Build history of the part. All positions in model axes, mm. A direction names the side the tool comes from. Coordinates: 2 decimals unless noted, no trailing zeros. Loops run counter-clockwise (first coordinate to the right, second up) from the corner with the lowest first, then second, coordinate; pieces in that order, holes last.
(1) Tool access for faces 5 (the face through (-7, -80, 12)), 6 (the face through (-26, -39.169, 12)), 7 (the face through (-13, -75, 12)): list every direction of +Z, -Z, +X, -X, +Y, -Y with a clear straight run to the whole face (end or side of a thin tool).
(2) Flat gauge pins, fed straight in: P1, Ø1, axis at y = -14, z = 15.5, coming from the +X side; P2, Ø11.5, axis at y = -76.5, z = 9, coming from the -X side; P3, Ø1, axis at x = -16, z = 14, coming from the -Y side; P4, Ø10, axis at x = -37.5, z = 4, coming from the -Y side. Where does each tip first touch, or does it go through?
(3) Slice it at A-A (z = 18.5). Give the number of separate pieces and of enclosed holes in the cut face, and give its area (3 significant figures).
(4) Wall check: L1, parallel to Y at x = -28, z = 23.25; L2, parallel to Y at x = -15.5, z = 7; L3, parallel to Y at x = -58.5, z = 4. Give the ranges that are in metal, low to high.
(5) Two-plate mould, pull along Y, no slides. Class faces 1 (the face through (-27.87, -31.5, 12.32)), 2 (the face through (-23.547, -29.477, 12.325)), 3 (the face through (-39, 0, 12)), 4 (the face through (0, -42, 12)): pulls with the +Y half, pulls with the -Y half, needs draft (parallel to the pull), parting line crosses it, or undercut.
(6) Slice it at B-B (y = -75). Give the cut face in (x, z), and give its area (3 significant figures).
(7) Slice it at C-C (x = -73). Give the cut face in (y, z).
from build123d import *

# Parameters (mm, degrees)
F1_DEPTH = 25
F3_DEPTH = 25


with BuildPart() as f1:
    # F0 (on Top) → F1 (new body)
    with BuildSketch(Plane.XY):
        with BuildLine():
            Line((0, -80), (0, -2))
            ThreePointArc((0, -2), (-0.5857864376, -0.5857864376), (-2, 0))
            Line((-2, 0), (-77.9695956579, 0))
            ThreePointArc((-77.9695956579, 0), (-79.3944371446, -0.5964948388), (-79.9693680385, -2.0301732624))
            Line((-79.9693680385, -2.0301732624), (-79.8235436371, -11.6948759406))
            ThreePointArc((-79.8235436371, -11.6948759406), (-79.2164881491, -13.1000910078), (-77.793597994, -13.6644750587))
            Line((-77.793597994, -13.6644750587), (-53.4198508516, -13.2967154695))
            add(Edge.make_bspline(
                [(-53.4198508516, -13.2967154695), (-47.7391326457, -13.5155175895), (-42.3810972533, -14.1065922457), (-38.542901615, -14.7899318492)],
                knots=[0, 0, 0, 0, 0.162253053, 0.162253053, 0.162253053, 0.162253053], degree=3))
            add(Edge.make_bspline(
                [(-38.542901615, -14.7899318492), (-35.6620781643, -15.3028240882), (-33.637457964, -15.8676938778), (-30.542901615, -17.425809837)],
                knots=[0.162253053, 0.162253053, 0.162253053, 0.162253053, 0.28403486, 0.28403486, 0.28403486, 0.28403486], degree=3))
            add(Edge.make_bspline(
                [(-30.542901615, -17.425809837), (-26.1822221976, -19.6214215586), (-19.6969808737, -23.7893126338), (-16.9190281723, -27.1281322878)],
                knots=[0.28403486, 0.28403486, 0.28403486, 0.28403486, 0.4556431162, 0.4556431162, 0.4556431162, 0.4556431162], degree=3))
            add(Edge.make_bspline(
                [(-16.9190281723, -27.1281322878), (-15.0709363906, -29.3493526709), (-14.8636375386, -31.2036378987), (-14.5838867171, -34.1526714679)],
                knots=[0.4556431162, 0.4556431162, 0.4556431162, 0.4556431162, 0.5698091378, 0.5698091378, 0.5698091378, 0.5698091378], degree=3))
            add(Edge.make_bspline(
                [(-14.5838867171, -34.1526714679), (-14.185393399, -38.3534461651), (-13.6398891789, -44.7755537277), (-13.3562185193, -49.1226911473)],
                knots=[0.5698091378, 0.5698091378, 0.5698091378, 0.5698091378, 0.7324338497, 0.7324338497, 0.7324338497, 0.7324338497], degree=3))
            add(Edge.make_bspline(
                [(-13.3562185193, -49.1226911473), (-13.1491946262, -52.2952480614), (-13.0816268013, -54.3626480299), (-13.0485558451, -57.1167729382)],
                knots=[0.7324338497, 0.7324338497, 0.7324338497, 0.7324338497, 0.851117964, 0.851117964, 0.851117964, 0.851117964], degree=3))
            add(Edge.make_bspline(
                [(-13.0485558451, -57.1167729382), (-13.0070703326, -60.5716558966), (-13.0198697257, -65.1071818251), (-13, -69.7056261365)],
                knots=[0.851117964, 0.851117964, 0.851117964, 0.851117964, 1, 1, 1, 1], degree=3))
            Line((-13, -69.7056261365), (-13, -80))
            Line((-13, -80), (0, -80))
        make_face()
        with BuildLine():
            add(Edge.make_bspline(
                [(-38.542901615, -14.7899318492), (-40.9139160013, -27.8005372261), (-38.6884407603, -47.6270350351), (-23.5400479968, -56.7981427702), (-13.0485558451, -57.1167729382)],
                knots=[0, 0, 0, 0, 0.5296598009, 1, 1, 1, 1], degree=3))
            Line((-13.0485558451, -57.1167729382), (-13.3562185193, -49.1226911473))
            add(Edge.make_bspline(
                [(-28.0948624921, -41.658554015), (-25.10242463, -46.0305335019), (-19.1761098596, -47.5514449335), (-13.3562185193, -49.1226911473)],
                knots=[0.5483675118, 0.5483675118, 0.5483675118, 0.5483675118, 1, 1, 1, 1], degree=3))
            add(Edge.make_bspline(
                [(-29.6557347838, -38.4299094695), (-29.4003822649, -39.4415698152), (-29.0648385357, -40.4727694453), (-28.0948624921, -41.658554015)],
                knots=[2.4430203601, 2.4430203601, 2.4430203601, 2.4430203601, 5.8501597635, 5.8501597635, 5.8501597635, 5.8501597635], degree=3))
            add(Edge.make_bspline(
                [(-30.1900775171, -36.4835122599), (-30.0399059836, -37.1596607946), (-29.863001925, -37.8096107603), (-29.6557347838, -38.4299094695)],
                knots=[0.399285872, 0.399285872, 0.399285872, 0.399285872, 0.4502459731, 0.4502459731, 0.4502459731, 0.4502459731], degree=3))
            add(Edge.make_bspline(
                [(-30.2856540448, -36.0319675746), (-30.2550717037, -36.1837342297), (-30.2232258771, -36.334261503), (-30.1900775171, -36.4835122599)],
                knots=[0.3880371104, 0.3880371104, 0.3880371104, 0.3880371104, 0.399285872, 0.399285872, 0.399285872, 0.399285872], degree=3))
            add(Edge.make_bspline(
                [(-30.542901615, -17.425809837), (-30.892076359, -24.086456269), (-31.3406220256, -30.7966273139), (-30.2856540448, -36.0319675746)],
                knots=[0, 0, 0, 0, 0.3880371104, 0.3880371104, 0.3880371104, 0.3880371104], degree=3))
            add(Edge.make_bspline(
                [(-38.542901615, -14.7899318492), (-35.6620781643, -15.3028240882), (-33.637457964, -15.8676938778), (-30.542901615, -17.425809837)],
                knots=[0.162253053, 0.162253053, 0.162253053, 0.162253053, 0.28403486, 0.28403486, 0.28403486, 0.28403486], degree=3))
        make_face()
        with BuildLine():
            Line((-13.3562185193, -49.1226911473), (-13.0485558451, -57.1167729382))
            add(Edge.make_bspline(
                [(-13.3562185193, -49.1226911473), (-13.1491946262, -52.2952480614), (-13.0816268013, -54.3626480299), (-13.0485558451, -57.1167729382)],
                knots=[0.7324338497, 0.7324338497, 0.7324338497, 0.7324338497, 0.851117964, 0.851117964, 0.851117964, 0.851117964], degree=3))
        make_face()
    extrude(amount=F1_DEPTH)

    # F2 (on Top) → F3 (join)
    with BuildSketch(Plane.XY):
        with BuildLine():
            Line((-25.0898172111, -30.0360443188), (-32.0051051676, -33.6804613471))
            Line((-32.0051051676, -33.6804613471), (-30.857918683, -39.1688235104))
            Line((-30.857918683, -39.1688235104), (-22.4874541369, -39.1688235104))
            ThreePointArc((-22.4874541369, -39.1688235104), (-20.9994273294, -38.981376841), (-19.6043757451, -38.4307489172))
            Line((-19.6043757451, -38.4307489172), (-12.428862974, -34.4991907477))
            Line((-12.428862974, -34.4991907477), (-13.2681293624, -29.8431319511))
            Line((-13.2681293624, -29.8431319511), (-21.9548307901, -29.3535438949))
            ThreePointArc((-21.9548307901, -29.3535438949), (-23.5687895254, -29.4813601163), (-25.0898172111, -30.0360443188))
        make_face()
        Polygon((-19.8781598252, -23.5392715438), (-23.3667287976, -19.8491029441), (-32.8251793981, -23.714505136), (-31.0336794844, -28.0982180313), align=None)
        Polygon((-11.7061119527, -40.9006923437), (-26.9871223718, -44.3079471588), (-25.5416221917, -48.8509498537), (-9.744361043, -45.3404448926), align=None)
    extrude(amount=F3_DEPTH)


solid = f1.part
Response values:
1. face 5: +Z, -Z, +X, -X, -Y
1. face 6: +Z, -Z
1. face 7: +Z, -Z, -X, -Y
2. P1: stops at x = 0
2. P2: stops at x = -13
2. P3: stops at y = -56.96
2. P4: stops at y = -49.01
3. separate pieces: 1
3. enclosed holes: 4
3. area: 2,800 mm2
4. L1: y = -52.85 to -41.79, -39.17 to -31.57, -26.86 to -21.74, -18.8 to 0
4. L2: y = -56.96 to -48.54, -46.62 to -41.75, -36.18 to -29.72, -29.41 to 0
4. L3: y = -13.37 to 0
5. face 1: undercut
5. face 2: undercut
5. face 3: pulls with the +Y half
5. face 4: needs draft
6. outline: (-13, 0) - (0, 0) - (0, 25) - (-13, 25) - close
6. area: 325 mm2
7. outline: (-13.59, 0) - (0, 0) - (0, 25) - (-13.59, 25) - close
